from build123d import *

# Parameters (mm, degrees)
SKETCH_1_W           = 20
SKETCH_1_H           = 10
EXTRUDE_1_DEPTH      = 10
EXTRUDE_2_DEPTH      = 3
EXTRUDE_2_DEPTH_BACK = 23
SKETCH_2_W           = 1
SKETCH_2_H           = 1
SKETCH_3_R           = 0.5
EXTRUDE_3_DEPTH      = 9


with BuildPart() as part:
    # Sketch 1 → Extrude 1 (new body)
    with BuildSketch(Plane.XY):
        with Locations((10, 5)):
            Rectangle(SKETCH_1_W, SKETCH_1_H)
    extrude(amount=EXTRUDE_1_DEPTH)

    # Sketch 2 → Extrude 2 (add, two sides: drawn at the far end of the back side and taken through both)
    with BuildSketch(Plane(origin=(20, 0, 0), x_dir=(0, 0, -1), z_dir=(1, 0, 0)).offset(-EXTRUDE_2_DEPTH_BACK)):
        with Locations((-5, 5)):
            Rectangle(SKETCH_2_W, SKETCH_2_H)
    extrude(amount=EXTRUDE_2_DEPTH + EXTRUDE_2_DEPTH_BACK)

    # Sketch 3 → Extrude 3 (add)
    with BuildSketch(Plane.XZ.offset(-4.5)):
        with Locations(Location((-2.5, 5, 0), (0, 0, 270))):
            Circle(SKETCH_3_R)
        with Locations(Location((22.5, 5, 0), (0, 0, 270))):
            Circle(SKETCH_3_R)
    extrude(amount=EXTRUDE_3_DEPTH)


solid = part.part
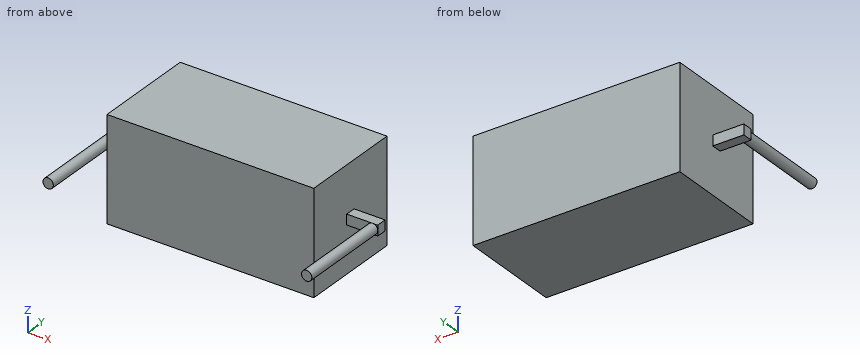
Input: part model. Units: mm. Frame: model coordinates. Round coordinates to 2 decimals unless told otherwise and drop trailing zeros. Loops run counter-clockwise (first coordinate to the right, second up) from the corner with the lowest first, then second, coordinate; pieces in that order, holes last. Notation, with made-up numbers: (0, 54) -> (5, 54) arc R22 ccw to (5, 75) -> close; hole circle Ø10 at (-10, -12). An arc over 180 degrees is marked (long way). Answer as a JSON object with one key per item and string values. Group by question number.
1) Section query B-B on y = 6. Output: boundary loops of the cut face in (x, z).
2) Ray query, L1, parallel to Y at x = 13, z = 8.5; L2, parallel to X at y = 7, z = 2.25; L3, parallel to X at y = 2.75, z = 4.75. Return the intervals inside material, ascending.
3) Pin query (flat end, axial travel): pin 1 (5 mm diameter, centred on x = 6.5, z = 5, fed in from -Y); pin 2 (1.1 mm diameter, centred on x = 21, y = 5, fed in from +Z); pin 3 (1.5 mm diameter, centred on y = 1, z = 8.5, fed in from +X). Return the tip coordinate at first contact, or that it passes through.
4) Section query A-A on y = 3.75. Output: boundary loops of the cut face in (x, z).
Reply:
{
 "1": {"outline": "(0, 0) -> (20, 0) -> (20, 10) -> (0, 10) -> close"},
 "2": {"L1": "y = 0 to 10", "L2": "x = 0 to 20", "L3": "x = -2.93 to -2.07, 0 to 20, 22.07 to 22.93"},
 "3": {"pin 1": "stops at y = 0", "pin 2": "stops at z = 5.5", "pin 3": "stops at x = 20"},
 "4": {"outline": "circle Ø1 at (-2.5, 5); (0, 0) -> (20, 0) -> (20, 10) -> (0, 10) -> close; circle Ø1 at (22.5, 5)"}
}
